Check sheet for the modelled part. Datum: model origin and axes. Units: mm. Round coordinates to 2 decimals unless told otherwise and drop trailing zeros. Write each loop counter-clockwise with the first axis right and the second up, starting at its lowest first coordinate (ties: lowest second). Pieces come first, ordered by that corner, then holes.
from build123d import *

# Parameters (mm, degrees)
BOSS_EXTRUDE1_DEPTH         = 6.35
SKETCH2_R                   = 2.5796875
SKETCH2_R_2                 = 3.175
CUT_EXTRUDE1_DEPTH          = 382.052912992
SKETCH3_R                   = 1.905
CUT_EXTRUDE2_DEPTH          = 382.052912992
F_1_4_20_TAPPED_HOLE1_D     = 5.1054
F_1_4_20_TAPPED_HOLE1_DEPTH = 16.51
F_1_4_20_TAPPED_HOLE1_TIP   = 1.533816902


with BuildPart() as part:
    # Sketch1 → Boss-Extrude1 (new body)
    with BuildSketch(Plane(origin=(0, 0, 0), x_dir=(1, 0, 0), z_dir=(0, 1, 0))):
        Polygon((0, 0), (228.6, 0), (228.6, 25.4), (133.35, 304.8), (95.25, 304.8), (0, 25.4), align=None)
    extrude(amount=BOSS_EXTRUDE1_DEPTH)

    # Sketch2 → Cut-Extrude1 (cut, through all)
    with BuildSketch(Plane(origin=(0, 6.35, 0), x_dir=(1, 0, 0), z_dir=(0, 1, 0))):
        with Locations(Location((165.1, 12.7, 0), (0, 0, 270))):
            Circle(SKETCH2_R)
        with Locations(Location((114.3, 12.7, 0), (0, 0, 270))):
            Circle(SKETCH2_R)
        with Locations(Location((63.5, 12.7, 0), (0, 0, 270))):
            Circle(SKETCH2_R)
        with Locations(Location((114.3, 38.1, 0), (0, 0, 270))):
            Circle(SKETCH2_R_2)
        with Locations(Location((114.3, 118.0846, 0), (0, 0, 270))):
            Circle(SKETCH2_R_2)
        with Locations(Location((114.3, 198.0692, 0), (0, 0, 270))):
            Circle(SKETCH2_R_2)
        with Locations(Location((114.3, 278.0538, 0), (0, 0, 270))):
            Circle(SKETCH2_R_2)
        with Locations(Location((12.7, 12.7, 0), (0, 0, 270))):
            Circle(SKETCH2_R)
        with Locations(Location((215.9, 12.7, 0), (0, 0, 270))):
            Circle(SKETCH2_R)
    extrude(amount=-CUT_EXTRUDE1_DEPTH, mode=Mode.SUBTRACT)

    # Sketch3 → Cut-Extrude2 (cut, through all)
    with BuildSketch(Plane(origin=(0, 6.35, 0), x_dir=(1, 0, 0), z_dir=(0, 1, 0))):
        with Locations(Location((133.35, 65.024, 0), (0, 0, 270))):
            Circle(SKETCH3_R)
        with Locations(Location((95.25, 65.024, 0), (0, 0, 270))):
            Circle(SKETCH3_R)
        with Locations(Location((133.35, 141.224, 0), (0, 0, 270))):
            Circle(SKETCH3_R)
        with Locations(Location((95.25, 141.224, 0), (0, 0, 270))):
            Circle(SKETCH3_R)
    extrude(amount=-CUT_EXTRUDE2_DEPTH, mode=Mode.SUBTRACT)

    # 1/4-20 Tapped Hole1
    with Locations(Plane(origin=(0, 6.35, 0), x_dir=(1, 0, 0), z_dir=(0, 1, 0))):
        with Locations((95.25, 141.224), (133.35, 141.224), (133.35, 65.024), (95.25, 65.024)):
            Hole(F_1_4_20_TAPPED_HOLE1_D / 2, depth=F_1_4_20_TAPPED_HOLE1_DEPTH)
            with Locations((0, 0, -(F_1_4_20_TAPPED_HOLE1_DEPTH + F_1_4_20_TAPPED_HOLE1_TIP / 2))):  # 118° drill point
                Cone(0, F_1_4_20_TAPPED_HOLE1_D / 2, F_1_4_20_TAPPED_HOLE1_TIP, mode=Mode.SUBTRACT)


solid = part.part
1. Release check for a two-part mould opening along Z. For faces 1 (the flat face through (113, 3, 0)), 2 (the cylindrical face through (112.37, 3.22, -200.59)), 3 (the flat face through (115, 3, -304.8)), 4 (the cylindrical face through (111.483, 3.219, -116.62)) record: released by +Z, released by -Z, zero draft, split by the parting line, or undercut.
2. Sectioned sample at A-A, the plane z = -38.1. Enter the section's corners in (x, y) (3 decimals), plus the area to 3 significant figures.
3. Scan lines: line 1 along X through (y, z) = (1.75, -12.7); line 2 along X through (y, z) = (2, -165.5); line 3 along X through (y, z) = (2.25, -41). Record each from-to range of solid material in increasing order.
4. Go/stop test with flat-tipped pins: pin 1 (4 mm diameter, centred on x = 95.25, z = -65.024, fed in from +Y); pin 2 (1.5 mm diameter, centred on y = 3, z = -150, fed in from -X). Record where each tip stops, or that it passes through.
5. Sectioned sample at D-D, the plane z = -214.5. Enter the section's corners in (x, y), plus the area to 3 significant figures.
6. Sectioned sample at C-C, the plane x = 180. Enter the section's corners in (y, z), plus the area to 3 significant figures.
7. Sectioned sample at B-B, the plane y = 3.5. Give the number of separate pieces and of enclosed holes in the cut face, plus the area to 3 significant figures.
Computed values:
1. face 1: released by +Z
1. face 2: undercut
1. face 3: released by -Z
1. face 4: undercut
2. outline: (4.33, 0) - (111.125, 0) - (111.125, 6.35) - (4.33, 6.35) - close; (117.475, 0) - (224.27, 0) - (224.27, 6.35) - (117.475, 6.35) - close
2. area: 1,360 mm2
3. line 1: x = 0 to 10.12, 15.28 to 60.92, 66.08 to 111.72, 116.88 to 162.52, 167.68 to 213.32, 218.48 to 228.6
3. line 2: x = 47.76 to 180.84
3. line 3: x = 5.32 to 113.01, 115.59 to 223.28
4. pin 1: passes through
4. pin 2: stops at x = 42.22
5. outline: (64.47, 0) - (164.13, 0) - (164.13, 6.35) - (64.47, 6.35) - close
5. area: 633 mm2
6. outline: (0, -167.96) - (6.35, -167.96) - (6.35, 0) - (0, 0) - close
6. area: 1,070 mm2
7. separate pieces: 1
7. enclosed holes: 13
7. area: 42,800 mm2
